```python
from build123d import *

# Parameters (mm, degrees)
CROQUIS1_W                    = 50.8
CROQUIS1_H                    = 25.4
CROQUIS1_W_2                  = 47.8
CROQUIS1_H_2                  = 22.4
SALIENTE_EXTRUIR1_DEPTH       = 450
CROQUIS2_R                    = 16
CORTAR_EXTRUIR1_DEPTH         = 26
TALADRO_DE_MARGEN_PARA_1_42_D = 6.7564
CROQUIS7_R                    = 6
CROQUIS7_R_2                  = 2.5
CORTAR_EXTRUIR2_DEPTH         = 25.4


with BuildPart() as part:
    # Croquis1 → Saliente-Extruir1 (new body)
    with BuildSketch(Plane.XY):
        Rectangle(CROQUIS1_W, CROQUIS1_H)
        Rectangle(CROQUIS1_W_2, CROQUIS1_H_2, mode=Mode.SUBTRACT)
    extrude(amount=SALIENTE_EXTRUIR1_DEPTH)

    # Croquis2 → Cortar-Extruir1 (cut)
    with BuildSketch(Plane(origin=(0, 12.7, 0), x_dir=(1, 0, 0), z_dir=(0, 1, 0))):
        with Locations((0, -387.5)):
            Circle(CROQUIS2_R)
    extrude(amount=-CORTAR_EXTRUIR1_DEPTH, mode=Mode.SUBTRACT)

    # Taladro de margen para 1/42 (through all)
    with Locations(Plane(origin=(-26.4, 572.488619806, 162.989101594), x_dir=(0, -1, 0), z_dir=(-1, 0, 0))):
        with Locations((572.888619806, 269.010898406), (572.888619806, 178.010898406), (572.888619806, 144.010898406)):
            Hole(TALADRO_DE_MARGEN_PARA_1_42_D / 2)

    # Croquis7 → Cortar-Extruir2 (cut)
    with BuildSketch(Plane(origin=(0, 12.7, 0), x_dir=(1, 0, 0), z_dir=(0, 1, 0))):
        with Locations((-14.9, -298.5)):
            Circle(CROQUIS7_R)
        with Locations((-14.9, -280.8)):
            Circle(CROQUIS7_R_2)
        with Locations((-14.9, -316.2)):
            Circle(CROQUIS7_R_2)
    extrude(amount=-CORTAR_EXTRUIR2_DEPTH, mode=Mode.SUBTRACT)


solid = part.part
```
Input: part model. Units: mm. Frame: model coordinates. A direction names the side the tool comes from. Round coordinates to 2 decimals unless told otherwise and drop trailing zeros. Loops run counter-clockwise (first coordinate to the right, second up) from the corner with the lowest first, then second, coordinate; pieces in that order, holes last. Notation, with made-up numbers: (30.25, -33) -> (52.25, -33) arc R17 ccw to (52.25, -7) -> close; hole circle Ø10 at (69.25, -34). An arc over 180 degrees is marked (long way). Use one line per item in the form item = value. Start each with the question number.
Item 1: Material intervals for L1, parallel to Z at x = 24.8, y = -0.4; L2, parallel to X at y = 10, z = 311.5; L3, parallel to X at y = -11.65, z = 316.2, sorted ascending. Write a range as from..to.
Item 2: Set-up query: faces 1 (the face through (0, -12.7, 222)), 2 (the face through (0, -11.2, 222)). Return all of +Z, -Z, +X, -X, +Y, -Y with unobstructed straight access to the full face (end or side cutting, diameter ignored); none if empty.
Item 3: Section query B-B on z = 74. Return the cut outline in (x, y), then the cut area to 3 significant figures.
Item 4: Section query A-A on z = 399. Return the cut outline in (x, y).
Item 5: Contact query for a flat-ended pin moving along its axis: pin 1 Ø6 at (y, z) = (-0.4, 432) entering from -X. Output: stop coordinate, or through.
Item 6: Mould query, pull axis Y, two halves, no side actions, for faces 3 (the face through (-23.9, 0, 222)), 4 (the face through (0, 11.2, 222)), 5 (the face through (0, -12, 0)), 6 (the face through (0, 12.7, 222)). Classes: pulls with the +Y half, pulls with the -Y half, needs draft (parallel to the pull), parting line crosses it, or undercut.
Ans:
q1.L1 = 0..303.62, 310.38..337.62, 344.38..428.62, 435.38..450
q1.L2 = -25.4..-23.9, 23.9..25.4
q1.L3 = -25.4..-17.4, -12.4..25.4
q2.face_1 = +Z, -Z, +X, -X, -Y
q2.face_2 = +Z, -Z
q3.outline = (-25.4, -12.7) -> (25.4, -12.7) -> (25.4, 12.7) -> (-25.4, 12.7) -> close; hole (-23.9, -11.2) -> (23.9, -11.2) -> (23.9, 11.2) -> (-23.9, 11.2) -> close
q3.area = 220 mm^2
q4.outline = (-25.4, -12.7) -> (-11.12, -12.7) -> (-11.12, -11.2) -> (-23.9, -11.2) -> (-23.9, 11.2) -> (-11.12, 11.2) -> (-11.12, 12.7) -> (-25.4, 12.7) -> close; (11.12, -12.7) -> (25.4, -12.7) -> (25.4, 12.7) -> (11.12, 12.7) -> (11.12, 11.2) -> (23.9, 11.2) -> (23.9, -11.2) -> (11.12, -11.2) -> close
q5.pin_1 = through
q6.face_3 = undercut
q6.face_4 = undercut
q6.face_5 = needs draft
q6.face_6 = pulls with the +Y half
